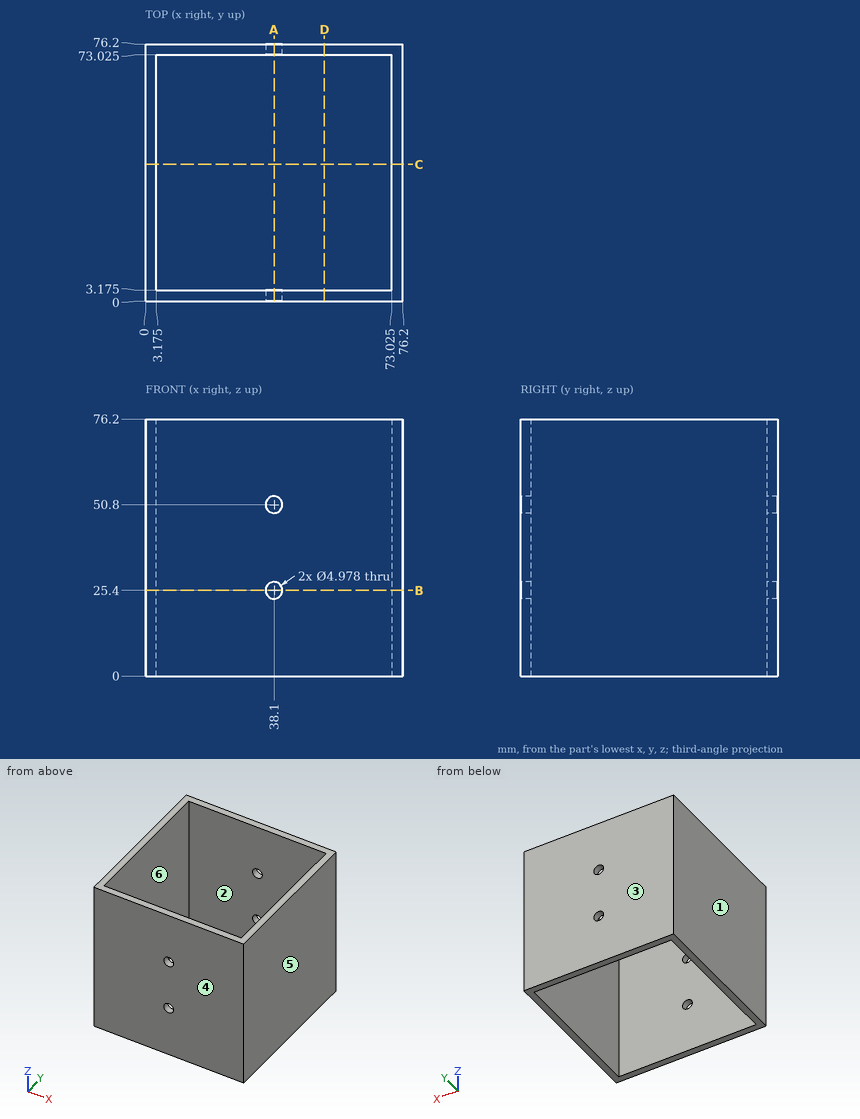
Answer from the drawing. Dimensions are ordinates in mm from the lowest x, y and z of the part. A direction names the side the tool comes from. Give positions to 0.01 mm unless a question says otherwise; leave off trailing zeros. Order: outer loops, then holes, each group sorted by start corner. A loop starts at its lowest first (then second) coordinate and runs counter-clockwise, first axis right, second up. Notation, with made-up numbers: (84, -25.5) -> (94, -25.5) arc R13 ccw to (94, -14.5) -> close; hole circle Ø7 at (78, 54.25). An arc over 180 degrees is marked (long way). One line per item, written item: value.
Item 1: Find section A-A, the plane x = 38.1. Give the vertices of the cut face in (y, z) (1 decimal).
Answer sheet:
outline: (0, 0) -> (3.2, 0) -> (3.2, 22.9) -> (0, 22.9) -> close; (0, 27.9) -> (3.2, 27.9) -> (3.2, 48.3) -> (0, 48.3) -> close; (0, 53.3) -> (3.2, 53.3) -> (3.2, 76.2) -> (0, 76.2) -> close; (73, 0) -> (76.2, 0) -> (76.2, 22.9) -> (73, 22.9) -> close; (73, 27.9) -> (76.2, 27.9) -> (76.2, 48.3) -> (73, 48.3) -> close; (73, 53.3) -> (76.2, 53.3) -> (76.2, 76.2) -> (73, 76.2) -> close
Item 2: Find section C-C, the plane y = 40.5. Give the vertices of the cut face in (x, z) (1 decimal).
Answer sheet:
outline: (0, 0) -> (3.2, 0) -> (3.2, 76.2) -> (0, 76.2) -> close; (73, 0) -> (76.2, 0) -> (76.2, 76.2) -> (73, 76.2) -> close
Item 3: Straight lines are drawn through the part: probe 1 along Z at (x, y) = (38.1, 1.25); probe 2 along Y at (x, z) = (16.5, 65.5) (1 decimal). For each, find the intervals that lie inside material, in ascending order.
Answer sheet:
probe 1: 0 to 22.91, 27.89 to 48.31, 53.29 to 76.2
probe 2: 0 to 3.2, 73 to 76.2
Item 4: A tool of negligible diameter and unlimited length cuts with its end or side. For the marked faces 5 and 6, from which of +Z, -Z, +X, -X, +Y, -Y can it reach the whole face along a straight path? Write none if from no direction.
Answer sheet:
face 5: +Z, -Z, +X, +Y, -Y
face 6: +Z, -Z
Item 5: Find section B-B, the plane z = 25.4. Give the vertices of the cut face in (x, y) (1 decimal).
Answer sheet:
outline: (0, 0) -> (35.6, 0) -> (35.6, 3.2) -> (3.2, 3.2) -> (3.2, 73) -> (35.6, 73) -> (35.6, 76.2) -> (0, 76.2) -> close; (40.6, 0) -> (76.2, 0) -> (76.2, 76.2) -> (40.6, 76.2) -> (40.6, 73) -> (73, 73) -> (73, 3.2) -> (40.6, 3.2) -> close
Item 6: Determine the mould class of the marked faces 1, 2, 3 and 4 for opening direction Y: released by +Y, released by -Y, zero draft, split by the parting line, or undercut.
Answer sheet:
face 1: zero draft
face 2: undercut
face 3: released by +Y
face 4: released by -Y
